Model file for the job. Use its own axes, mm. A direction names the side the tool comes from. Coordinates: 2 decimals unless noted, no trailing zeros. Order: outer loops, then holes, each group sorted by start corner. A loop starts at its lowest first (then second) coordinate and runs counter-clockwise, first axis right, second up. Notation, with made-up numbers: (66.25, -32.5) -> (121.25, -32.5) arc R18 ccw to (121.25, 1.5) -> close; hole circle Ø11 at (36.25, 66). An arc over 180 degrees is marked (long way). Use CSV: the item, a comma, the result in double quotes. Start each with the question number.
(1) Cut at A-A on y = -2.15. Give the number of separate pieces and of enclosed holes in the cut face, plus the area to 3 significant figures.
(2) Probe L1, parallel to X at y = -0.8, z = -32.5; L2, parallel to Z at x = -7, y = -1. List the from-to ranges inside material, lowest first.
(3) Cut at B-B on x = -5. Write the cut outline in (y, z), plus the area to 3 significant figures.
(4) Pull direction Z, two halves, no side cores. Call faces 1 (the flat face through (0, 0, 1)), 2 (the flat face through (12, -2, -65)), 3 (the flat face through (9, -2, 74.5)): pulls with the +Z half, pulls with the -Z half, needs draft (parallel to the pull), parting line crosses it, or undercut.
(5) Tool access for faces 4 (the flat face through (0, -3.048, 1)), 5 (the flat face through (12, -2, 55)), 6 (the flat face through (2, -2, -73)), 7 (the flat face through (9, -2, -74.5)), 8 (the flat face through (-8, -2, 73)): list every direction of +Z, -Z, +X, -X, +Y, -Y with a clear straight run to the whole face (end or side of a thin tool).
(6) Pin check, flat tip, straight feed: pin 1 Ø0.9 at (x, y) = (-1.5, -1) entering from +Z. Stop position of the tip, or through.
```python
from build123d import *

# Parameters (mm, degrees)
F0_W     = 2.999994
F0_H     = 10.000005
F0_H_2   = 9.99998
F1_DEPTH = 3.048


with BuildPart() as f1:
    # F0 (on Front) → F1 (new body)
    with BuildSketch(Plane.XZ):
        Polygon((16.499992, 74.500003), (1.999996, 74.500003), (1.999996, 71.500009), (-8.000009, 71.500009), (-8.000009, 74.500003), (-16.499992, 74.500003), (-16.499992, -74.499978), (-8.000009, -74.499978), (-8.000009, -71.499984), (1.999996, -71.499984), (1.999996, -74.499978), (16.499992, -74.499978), align=None)
        with Locations((12.000001, -59.999994)):
            Rectangle(F0_W, F0_H, mode=Mode.SUBTRACT)
        with Locations((12.000001, -29.999991)):
            Rectangle(F0_W, F0_H_2, mode=Mode.SUBTRACT)
        with Locations((12.000001, 1.2e-05)):
            Rectangle(F0_W, F0_H, mode=Mode.SUBTRACT)
        with Locations((12.000001, 30.000003)):
            Rectangle(F0_W, F0_H, mode=Mode.SUBTRACT)
        with Locations((12.000001, 60.000007)):
            Rectangle(F0_W, F0_H_2, mode=Mode.SUBTRACT)
    extrude(amount=F1_DEPTH)


solid = f1.part
```
Outcome:
1,separate pieces,"1"
1,enclosed holes,"5"
1,area,"4,710 mm2"
2,L1,"-16.5 to 10.5, 13.5 to 16.5"
2,L2,"-71.5 to 71.5"
3,outline,"(-3.05, -71.5) -> (0, -71.5) -> (0, 71.5) -> (-3.05, 71.5) -> close"
3,area,"436 mm2"
4,face 1,"needs draft"
4,face 2,"undercut"
4,face 3,"pulls with the +Z half"
5,face 4,"+Z, -Z, +X, -X, -Y"
5,face 5,"+Y, -Y"
5,face 6,"-Z, +Y, -Y"
5,face 7,"-Z, +X, -X, +Y, -Y"
5,face 8,"+Z, +Y, -Y"
6,pin 1,"z = 71.5"
